Design review of the part shown in the three views and the two pictorial views. Dimensions are in mm from the part's minimum x, y and z. Give positions to 0.01 mm unless a question says otherwise; leave off trailing zeros. Loops run counter-clockwise (first coordinate to the right, second up) from the corner with the lowest first, then second, coordinate; pieces in that order, holes last. Notation, with made-up numbers: (33, 72) - (55, 72) arc R23 ccw to (55, 105) - close; hole circle Ø2 at (86.25, 83.25). An arc over 180 degrees is marked (long way). Answer in a Markdown table with one row per item.
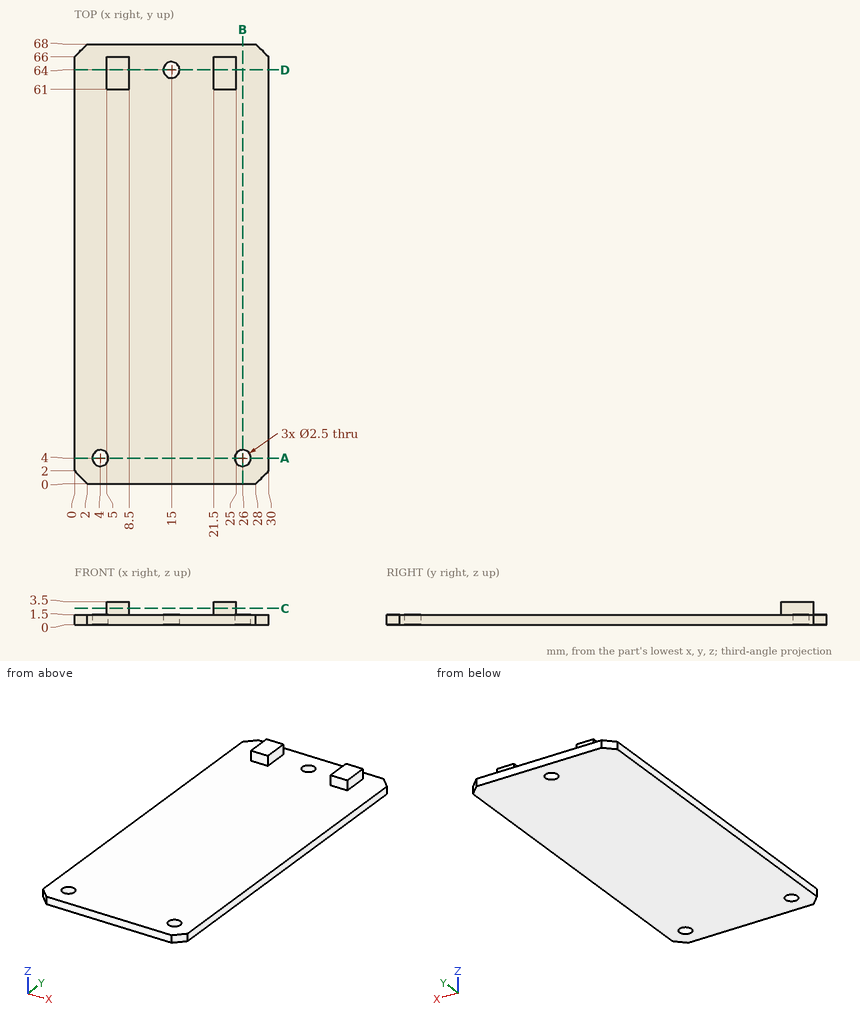
1. We need section D-D, the plane y = 64. Give the boundary of the cut face in (x, z).
Values:
| item | result |
|---|---|
| outline | (0, 0) - (13.75, 0) - (13.75, 1.5) - (8.5, 1.5) - (8.5, 3.5) - (5, 3.5) - (5, 1.5) - (0, 1.5) - close; (16.25, 0) - (30, 0) - (30, 1.5) - (25, 1.5) - (25, 3.5) - (21.5, 3.5) - (21.5, 1.5) - (16.25, 1.5) - close |
2. We need section A-A, the plane y = 4. Give the boundary of the cut face in (x, z).
Values:
| item | result |
|---|---|
| outline | (0, 0) - (2.75, 0) - (2.75, 1.5) - (0, 1.5) - close; (5.25, 0) - (24.75, 0) - (24.75, 1.5) - (5.25, 1.5) - close; (27.25, 0) - (30, 0) - (30, 1.5) - (27.25, 1.5) - close |
3. We need section C-C, the plane z = 2.5. Give the boundary of the cut face in (x, y), and give its area (3 significant figures).
Values:
| item | result |
|---|---|
| outline | (5, 61) - (8.5, 61) - (8.5, 66) - (5, 66) - close; (21.5, 61) - (25, 61) - (25, 66) - (21.5, 66) - close |
| area | 35.0 mm^2 |
4. We need section B-B, the plane x = 26. Give the boundary of the cut face in (y, z), and give its area (4 significant figures).
Values:
| item | result |
|---|---|
| outline | (0, 0) - (2.75, 0) - (2.75, 1.5) - (0, 1.5) - close; (5.25, 0) - (68, 0) - (68, 1.5) - (5.25, 1.5) - close |
| area | 98.25 mm^2 |
5. Wall thickness on line 1 (X direction, y = 64, z = 0.5); line 2 (Y direction, x = 15, z = 0.9); line 3 (Y direction, x = 26, z = 0.65): over which ranges is each line inside the solid? List them lowest first. Write a range as [from, to].
Values:
| item | result |
|---|---|
| line 1 | x = [0, 13.75], [16.25, 30] |
| line 2 | y = [0, 62.75], [65.25, 68] |
| line 3 | y = [0, 2.75], [5.25, 68] |
6. Clearance check with flat-ended pins moving along their axes: pin 1 (0.6 mm diameter, centred on y = 64, z = 2.5, fed in from +X); pin 2 (1.5 mm diameter, centred on x = 14.5, z = 2.5, fed in from +Y); pin 3 (3 mm diameter, centred on x = 15, y = 64, fed in from -Z); pin 4 (0.6 mm diameter, centred on x = 7, z = 3, fed in from +Y). State where each tip first meets the part, or that it passes through.
Values:
| item | result |
|---|---|
| pin 1 | stops at x = 25 |
| pin 2 | passes through |
| pin 3 | stops at z = 0 |
| pin 4 | stops at y = 66 |
